For this review, use the dimensioned drawing (mm, ordinates from the lowest corner) and the shaded views. A direction names the side the tool comes from. Coordinates: 2 decimals unless noted, no trailing zeros. Write each loop counter-clockwise with the first axis right and the second up, starting at its lowest first coordinate (ties: lowest second). Pieces come first, ordered by that corner, then holes. Notation, with made-up numbers: (12, 6.25) - (60, 6.25) arc R13 cw to (60, 24.25) - close; hole circle Ø11 at (2, 23.25). An arc over 180 degrees is marked (long way). One line per item, written item: value.
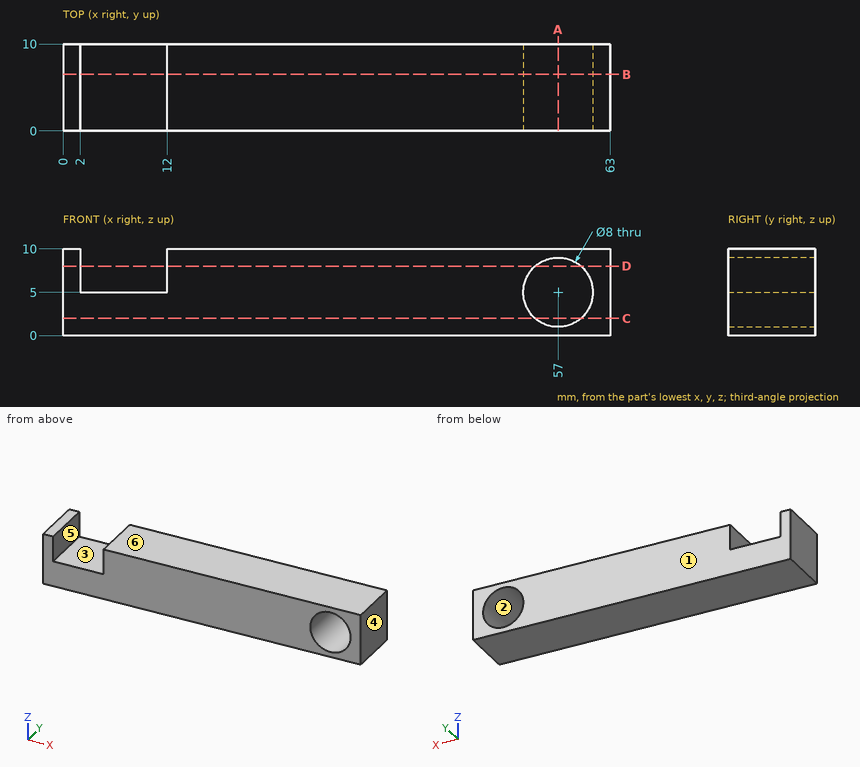
1. Consider section B-B, the plane y = 6.5. Write out the cut boundary in (x, z).
Answer block:
outline: (0, 0) - (63, 0) - (63, 10) - (12, 10) - (12, 5) - (2, 5) - (2, 10) - (0, 10) - close; hole circle Ø8 at (57, 5)
2. Consider section C-C, the plane z = 2. Write out the cut boundary in (x, y).
Answer block:
outline: (0, 0) - (54.35, 0) - (54.35, 10) - (0, 10) - close; (59.65, 0) - (63, 0) - (63, 10) - (59.65, 10) - close
3. Consider section A-A, the plane x = 57. Write out the cut boundary in (y, z).
Answer block:
outline: (0, 0) - (10, 0) - (10, 1) - (0, 1) - close; (0, 9) - (10, 9) - (10, 10) - (0, 10) - close
4. Consider section D-D, the plane z = 8. Write out the cut boundary in (x, y).
Answer block:
outline: (0, 0) - (2, 0) - (2, 10) - (0, 10) - close; (12, 0) - (54.35, 0) - (54.35, 10) - (12, 10) - close; (59.65, 0) - (63, 0) - (63, 10) - (59.65, 10) - close
5. For the marked faces 5 and 6, list the 3-axis set-ups (+Z, -Z, +X, -X, +Y, -Y) from which the entire face can be reached by the end or side of a thin tool; tool diameter is ignored.
Answer block:
face 5: +Z, +Y, -Y
face 6: +Z, +X, -X, +Y, -Y
6. Mouldability with a two-part tool opening along X and no side actions: class the marked faces 1, 2, 3 and 4 as released by +X, released by -X, zero draft, split by the parting line, or undercut.
Answer block:
face 1: zero draft
face 2: undercut
face 3: undercut
face 4: released by +X
7. Wall thickness on line 1 along Z through (x, y) = (57, 7.25); line 2 along X through (y, z) = (7, 7.25); line 3 along X through (y, z) = (3.75, 7): over which ranges is each line inside the solid? List them lowest first.
Answer block:
line 1: z = 0 to 1, 9 to 10
line 2: x = 0 to 2, 12 to 53.69, 60.31 to 63
line 3: x = 0 to 2, 12 to 53.54, 60.46 to 63
8. Insertion check: pin 1 Ø5.5 at (y, z) = (5, 8.5) entering from -X. The pin has a flat end and moves straight along its axis. Give the tip position at first contact, or say it passes through.
Answer block:
pin 1: stops at x = 0
